Part model, mm, in its own coordinate system. A direction names the side the tool comes from. Round coordinates to 2 decimals unless told otherwise and drop trailing zeros. Loops run counter-clockwise (first coordinate to the right, second up) from the corner with the lowest first, then second, coordinate; pieces in that order, holes last.
from build123d import *

# Parameters (mm, degrees)
SKETCH1_W           = 75.17
SKETCH1_H           = 67.47
SKETCH1_W_2         = 10.58
SKETCH1_H_2         = 22.218316852
BOSS_EXTRUDE1_DEPTH = 3.175
SKETCH2_R           = 1.415
CUT_EXTRUDE1_DEPTH  = 10


with BuildPart() as part:
    # Sketch1 → Boss-Extrude1 (new body)
    with BuildSketch(Plane.XY):
        Rectangle(SKETCH1_W, SKETCH1_H)
        with Locations((0, 14.675)):
            Rectangle(SKETCH1_W_2, SKETCH1_H_2, mode=Mode.SUBTRACT)
        with Locations((0, -14.675)):
            Rectangle(SKETCH1_W_2, SKETCH1_H_2, mode=Mode.SUBTRACT)
    extrude(amount=BOSS_EXTRUDE1_DEPTH)

    # Sketch2 → Cut-Extrude1 (cut)
    with BuildSketch(Plane.XY.offset(3.175)):
        with Locations((0, 30.553019485)):
            Circle(SKETCH2_R)
        with Locations((0, -30.553019485)):
            Circle(SKETCH2_R)
    extrude(amount=-CUT_EXTRUDE1_DEPTH, mode=Mode.SUBTRACT)


solid = part.part
1) Slice it at C-C, the plane z = 0.95. Give the cut face in (x, y) (3 decimals), then the cut area to 3 significant figures.
Values:
outline: (-37.585, -33.735) - (37.585, -33.735) - (37.585, 33.735) - (-37.585, 33.735) - close; hole (-5.29, -25.784) - (5.29, -25.784) - (5.29, -3.566) - (-5.29, -3.566) - close; hole (-5.29, 3.566) - (5.29, 3.566) - (5.29, 25.784) - (-5.29, 25.784) - close; hole circle Ø2.83 at (0, -30.553); hole circle Ø2.83 at (0, 30.553)
area: 4,590 mm2
2) Slice it at A-A, the plane x = 0. Give the cut face in (y, z) (3 decimals).
Values:
outline: (-33.735, 0) - (-31.968, 0) - (-31.968, 3.175) - (-33.735, 3.175) - close; (-29.138, 0) - (-25.784, 0) - (-25.784, 3.175) - (-29.138, 3.175) - close; (-3.566, 0) - (3.566, 0) - (3.566, 3.175) - (-3.566, 3.175) - close; (25.784, 0) - (29.138, 0) - (29.138, 3.175) - (25.784, 3.175) - close; (31.968, 0) - (33.735, 0) - (33.735, 3.175) - (31.968, 3.175) - close
3) Slice it at B-B, the plane y = -12.5. Give the cut face in (x, z) (3 decimals).
Values:
outline: (-37.585, 0) - (-5.29, 0) - (-5.29, 3.175) - (-37.585, 3.175) - close; (5.29, 0) - (37.585, 0) - (37.585, 3.175) - (5.29, 3.175) - close
4) Wall check: line 1 along Y through (x, z) = (0, 2.2) (3 decimals); line 2 along Y through (x, z) = (3.5, 1.35) (3 decimals); line 3 along X through (y, z) = (-22, 1.35) (3 decimals). Give the ranges that are in metal, low to high.
Values:
line 1: y = -33.735 to -31.968, -29.138 to -25.784, -3.566 to 3.566, 25.784 to 29.138, 31.968 to 33.735
line 2: y = -33.735 to -25.784, -3.566 to 3.566, 25.784 to 33.735
line 3: x = -37.585 to -5.29, 5.29 to 37.585
5) Mould opens along X. For faces 1 (the face through (-1, -33.735, 2)), 2 (the face through (0, -3.566, 2)), 3 (the face through (-37.585, 0, 2)) say: released by +X, released by -X, zero draft, split by the parting line, or undercut.
Values:
face 1: zero draft
face 2: undercut
face 3: released by -X
6) Tool access for faces 4 (the face through (5.29, -15, 2)), 5 (the face through (37.585, 0, 2)): list every direction of +Z, -Z, +X, -X, +Y, -Y with a clear straight run to the whole face (end or side of a thin tool).
Values:
face 4: +Z, -Z
face 5: +Z, -Z, +X, +Y, -Y
